Source: CAD feature listing. Evaluate the final solid. Frame: model axes, mm. Face numbers are marked on the shaded views. A direction names the side the tool comes from. Coordinates: 2 decimals unless noted, no trailing zeros. Loops run counter-clockwise (first coordinate to the right, second up) from the corner with the lowest first, then second, coordinate; pieces in that order, holes last. Notation, with made-up numbers: (32, -36) -> (69, -36) arc R18 ccw to (69, -17) -> close; hole circle Ø6 at (18, 53.5). An arc over 180 degrees is marked (long way). Answer as a JSON object with one key per item and string values. Group by question number.
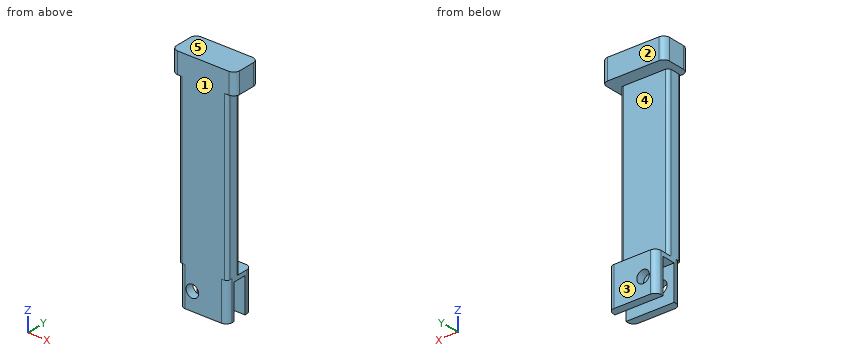
from build123d import *

# Parameters (mm, degrees)
F_01_START                                = 13
F_01_TPU_16_BY_5_GAUGE_DEPTH              = 55
F_02_CORD_END_BLOCK_DEPTH                 = 13
F_03_START                                = 68
F_03_CAPTURED_TAIL_BUTTON_DEPTH           = 7
F_04_START                                = -0.2
S04_OPEN_TWO_EAR_PIN_CLEVIS_W             = 18
S04_OPEN_TWO_EAR_PIN_CLEVIS_H             = 4.5
F_04_OPEN_TWO_EAR_PIN_CLEVIS_DEPTH        = 11.8
F_05_START                                = -5.2
S05_SHOULDER_PIN_THROUGH_BOTH_EARS_R      = 2.08
F_05_SHOULDER_PIN_THROUGH_BOTH_EARS_DEPTH = 10.4


with BuildPart() as part:
    # S01 - TPU 16 by 5 gauge → 01 - TPU 16 by 5 gauge (new body)
    with BuildSketch(Plane.XY.offset(F_01_START)):
        with BuildLine():
            Line((-7, -5), (7, -5))
            ThreePointArc((7, -5), (7.707106781, -4.707106781), (8, -4))
            Line((8, -4), (8, -1))
            ThreePointArc((8, -1), (7.707106781, -0.292893219), (7, 0))
            Line((7, 0), (-7, 0))
            ThreePointArc((-7, 0), (-7.707106781, -0.292893219), (-8, -1))
            Line((-8, -1), (-8, -4))
            ThreePointArc((-8, -4), (-7.707106781, -4.707106781), (-7, -5))
        make_face()
    extrude(amount=F_01_TPU_16_BY_5_GAUGE_DEPTH)

    # S02 - Cord end block → 02 - Cord end block (add)
    with BuildSketch(Plane.XY):
        with BuildLine():
            Line((-6, -5), (6, -5))
            ThreePointArc((6, -5), (7.414213562, -4.414213562), (8, -3))
            Line((8, -3), (8, 3))
            ThreePointArc((8, 3), (7.414213562, 4.414213562), (6, 5))
            Line((6, 5), (-6, 5))
            ThreePointArc((-6, 5), (-7.414213562, 4.414213562), (-8, 3))
            Line((-8, 3), (-8, -3))
            ThreePointArc((-8, -3), (-7.414213562, -4.414213562), (-6, -5))
        make_face()
    extrude(amount=F_02_CORD_END_BLOCK_DEPTH)

    # S03 - Captured tail button → 03 - Captured tail button (add)
    with BuildSketch(Plane.XY.offset(F_03_START)):
        with BuildLine():
            Line((-8.5, -5), (8.5, -5))
            ThreePointArc((8.5, -5), (9.914213562, -4.414213562), (10.5, -3))
            Line((10.5, -3), (10.5, 2.6))
            ThreePointArc((10.5, 2.6), (9.914213562, 4.014213562), (8.5, 4.6))
            Line((8.5, 4.6), (-8.5, 4.6))
            ThreePointArc((-8.5, 4.6), (-9.914213562, 4.014213562), (-10.5, 2.6))
            Line((-10.5, 2.6), (-10.5, -3))
            ThreePointArc((-10.5, -3), (-9.914213562, -4.414213562), (-8.5, -5))
        make_face()
    extrude(amount=F_03_CAPTURED_TAIL_BUTTON_DEPTH)

    # S04 - Open two-ear pin clevis → 04 - Open two-ear pin clevis (cut)
    with BuildSketch(Plane.XY.offset(F_04_START)):
        Rectangle(S04_OPEN_TWO_EAR_PIN_CLEVIS_W, S04_OPEN_TWO_EAR_PIN_CLEVIS_H)
    extrude(amount=F_04_OPEN_TWO_EAR_PIN_CLEVIS_DEPTH, mode=Mode.SUBTRACT)

    # S05 - Shoulder pin through both ears → 05 - Shoulder pin through both ears (cut)
    with BuildSketch(Plane(origin=(0, 0, 0), x_dir=(1, 0, 0), z_dir=(0, 1, 0)).offset(F_05_START)):
        with Locations(Location((-3.6, -6, 0), (0, 0, 90))):
            Circle(S05_SHOULDER_PIN_THROUGH_BOTH_EARS_R)
    extrude(amount=F_05_SHOULDER_PIN_THROUGH_BOTH_EARS_DEPTH, mode=Mode.SUBTRACT)


solid = part.part
1. Reachability of the marked faces 1 and 2 from +Z, -Z, +X, -X, +Y, -Y: full face, straight path, thin tool, end or side. Return the list, or none.
2. Mould query, pull axis Z, two halves, no side actions, for the marked faces 3, 4 and 5. Classes: pulls with the +Z half, pulls with the -Z half, needs draft (parallel to the pull), parting line crosses it, or undercut.
3. Section query A-A on z = 6. Return loops of the section in (x, y).
4. Section query B-B on x = -3.6. Return loops of the section in (y, z), then the cut area to 3 significant figures.
5. Ray query, L1, parallel to Z at x = 6.75, y = 1.5; L2, parallel to Z at x = -5.5, y = 3; L3, parallel to X at y = -2.9, z = 6. Return the intervals inside material, ascending.
6. Pin query (flat end, axial travel): pin 1 Ø8 at (x, z) = (3.5, 40) entering from +Y; pin 2 Ø1.3 at (x, y) = (-3.5, 0) entering from -Z; pin 3 Ø3.5 at (x, z) = (-0.5, 70.5) entering from +Y. Return the tip coordinate at first contact, or that it passes through.
7. Section query C-C on x = 5. Return loops of the section in (y, z).
8. Section query D-D on z = 69.5. Return loops of the section in (x, y), then the cut area to 3 significant figures.
Solved:
{
 "1": {"face 1": "+Z, -Z, +X, -X, -Y", "face 2": "+Z, +X, -X, +Y"},
 "2": {"face 3": "needs draft", "face 4": "undercut", "face 5": "pulls with the +Z half"},
 "3": {"outline": "(-8, -3) arc R2 ccw to (-6, -5) -> (-5.68, -5) -> (-5.68, -2.25) -> (-8, -2.25) -> close; (-8, 2.25) -> (-5.68, 2.25) -> (-5.68, 5) -> (-6, 5) arc R2 ccw to (-8, 3) -> close; (-1.52, -5) -> (6, -5) arc R2 ccw to (8, -3) -> (8, -2.25) -> (-1.52, -2.25) -> close; (-1.52, 2.25) -> (8, 2.25) -> (8, 3) arc R2 ccw to (6, 5) -> (-1.52, 5) -> close"},
 "4": {"outline": "(-5, 0) -> (-2.25, 0) -> (-2.25, 3.92) -> (-5, 3.92) -> close; (-5, 8.08) -> (-2.25, 8.08) -> (-2.25, 11.6) -> (2.25, 11.6) -> (2.25, 8.08) -> (5, 8.08) -> (5, 13) -> (0, 13) -> (0, 68) -> (4.6, 68) -> (4.6, 75) -> (-5, 75) -> close; (2.25, 0) -> (5, 0) -> (5, 3.92) -> (2.25, 3.92) -> close", "area": "397 mm^2"},
 "5": {"L1": "11.6 to 13, 68 to 75", "L2": "0 to 5.15, 6.85 to 13, 68 to 75", "L3": "-8 to -5.68, -1.52 to 8"},
 "6": {"pin 1": "y = 0", "pin 2": "z = 11.6", "pin 3": "y = 4.6"},
 "7": {"outline": "(-5, 0) -> (-2.25, 0) -> (-2.25, 11.6) -> (2.25, 11.6) -> (2.25, 0) -> (5, 0) -> (5, 13) -> (0, 13) -> (0, 68) -> (4.6, 68) -> (4.6, 75) -> (-5, 75) -> close"},
 "8": {"outline": "(-10.5, -3) arc R2 ccw to (-8.5, -5) -> (8.5, -5) arc R2 ccw to (10.5, -3) -> (10.5, 2.6) arc R2 ccw to (8.5, 4.6) -> (-8.5, 4.6) arc R2 ccw to (-10.5, 2.6) -> close", "area": "198 mm^2"}
}
